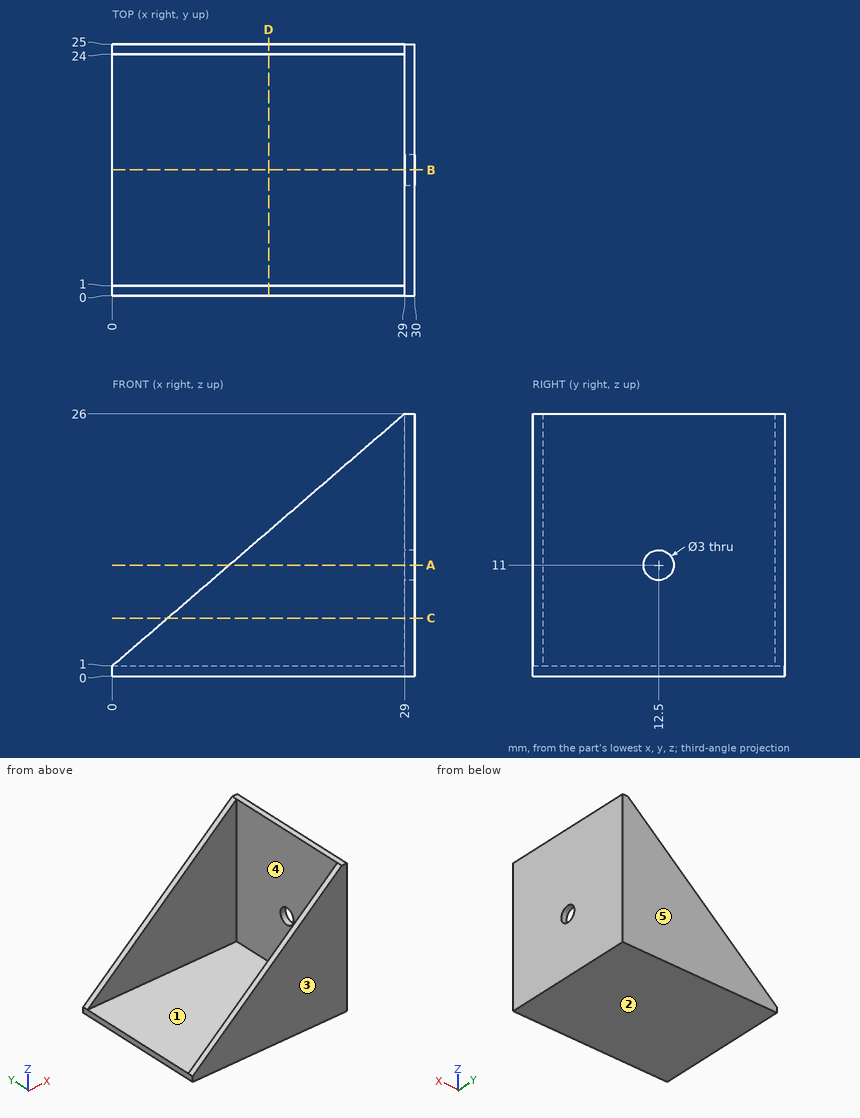
The drawing under review shows one solid part. Ordinate dimensions are in mm from its lowest x, y, z. A direction names the side the tool comes from. Coordinates: 2 decimals unless noted, no trailing zeros. Write each loop counter-clockwise with the first axis right and the second up, starting at its lowest first coordinate (ties: lowest second). Pieces come first, ordered by that corner, then holes. Notation, with made-up numbers: (75.5, -25) - (79.5, -25) arc R16 ccw to (79.5, 2) - close; hole circle Ø11 at (85, 24). An arc over 180 degrees is marked (long way). Use one line per item in the form item = value.
Q1. Consider section A-A (z = 11). Write out the cut boundary in (x, y), plus the area to 3 significant figures.
Taken from the geometry:
outline = (11.6, 0) - (30, 0) - (30, 11) - (29, 11) - (29, 1) - (11.6, 1) - close; (11.6, 24) - (29, 24) - (29, 14) - (30, 14) - (30, 25) - (11.6, 25) - close
area = 56.8 mm^2
Q2. Consider section C-C (z = 5.75). Write out the cut boundary in (x, y).
Taken from the geometry:
outline = (5.51, 0) - (30, 0) - (30, 25) - (5.51, 25) - (5.51, 24) - (29, 24) - (29, 1) - (5.51, 1) - close
Q3. Insertion check: pin 1 Ø3.5 at (y, z) = (12.5, 11) entering from -X; pin 2 Ø1 at (x, y) = (7.5, 17) entering from +Z. Each pin has a flat end and moves straight along its axis. Give the tip position at first contact, or say it passes through.
Taken from the geometry:
pin_1 = 29
pin_2 = 1
Q4. Machinability: for the marked faces 4 and 5, which of the approach directions +Z, -Z, +X, -X, +Y, -Y give a long, thin tool a straight path to every point of the face, cutting with its end or side? Answer none if there is none.
Taken from the geometry:
face_4 = +Z, -X
face_5 = +Z, -Z, +X, -X, +Y
Q5. Consider section D-D (x = 15.5). Write out the cut boundary in (y, z), plus the area to 3 significant figures.
Taken from the geometry:
outline = (0, 0) - (25, 0) - (25, 14.36) - (24, 14.36) - (24, 1) - (1, 1) - (1, 14.36) - (0, 14.36) - close
area = 51.7 mm^2
Q6. For probe 1 along Z at (x, y) = (29.5, 12.5); probe 2 along Y at (x, z) = (24.75, 17); probe 3 along X at (y, z) = (18.5, 10.5), list the stretches that pass through material, from the lowest coordinate up.
Taken from the geometry:
probe_1 = 0 to 9.5, 12.5 to 26
probe_2 = 0 to 1, 24 to 25
probe_3 = 29 to 30
Q7. The part is to be moulded in two halves that separate along Y. For the marked faces 1, 2 and 3, say which applies: +Y half, -Y half, draft (parallel to the pull), parting line (faces both ways), or undercut.
Taken from the geometry:
face_1 = undercut
face_2 = draft
face_3 = -Y half
Q8. Consider section B-B (y = 12.5). Write out the cut boundary in (x, z).
Taken from the geometry:
outline = (0, 0) - (30, 0) - (30, 9.5) - (29, 9.5) - (29, 1) - (0, 1) - close; (29, 12.5) - (30, 12.5) - (30, 26) - (29, 26) - close
